Can you work these out from the model? Positions are in its coordinate system, mm. Coordinates: 2 decimals unless noted, no trailing zeros. Order: outer loops, then holes, each group sorted by start corner. A loop starts at its lowest first (then second) coordinate and runs counter-clockwise, first axis right, second up.
```python
from build123d import *

# Parameters (mm, degrees)
SKETCH3_R          = 20.5
SKETCH3_R_2        = 1.5875
EXTRUDE2_DEPTH     = 0.1778
SKETCH5_R          = 1.5
CUT_EXTRUDE1_DEPTH = 29.991923235
CIRPATTERN1_COUNT  = 3


with BuildPart() as part:
    # Sketch3 → Extrude2 (new body)
    with BuildSketch(Plane.XY):
        Circle(SKETCH3_R)
        with Locations((0, 16.5)):
            Circle(SKETCH3_R_2, mode=Mode.SUBTRACT)
        with Locations((14.289419162, -8.25)):
            Circle(SKETCH3_R_2, mode=Mode.SUBTRACT)
        with Locations((-14.289419162, -8.25)):
            Circle(SKETCH3_R_2, mode=Mode.SUBTRACT)
    extrude(amount=EXTRUDE2_DEPTH)

    # Sketch5 → Cut-Extrude1 (cut, through all)
    with BuildSketch(Plane.XY):
        with BuildLine():
            Line((1.5, -20.4450483), (1.5, -16.5))
            ThreePointArc((1.5, -16.5), (0, -18), (-1.5, -16.5))
            Line((-1.5, -16.5), (-1.5, -20.4450483))
            ThreePointArc((-1.5, -20.4450483), (0, -20.5), (1.5, -20.4450483))
        make_face()
        with Locations((0, -16.5)):
            Circle(SKETCH5_R)
    cut_extrude1 = extrude(amount=CUT_EXTRUDE1_DEPTH, mode=Mode.SUBTRACT)

    # CirPattern1: Cut-Extrude1 ×3 about axis, 1 skipped
    cirpattern1_axis = Axis((0, 0, 0.1778), (0, 0, -1))
    add([cut_extrude1.rotate(cirpattern1_axis, i * 360 / CIRPATTERN1_COUNT) for i in range(1, CIRPATTERN1_COUNT) if i not in (1,)], mode=Mode.SUBTRACT)


solid = part.part
```
1. Imagine slicing it at B-B on z = 0.1. Give the number of separate pieces and of enclosed holes in the cut face, then the cut area to 3 significant figures.
Completed:
separate pieces: 1
enclosed holes: 3
area: 1,270 mm2
2. I'm going to push a flat-ended pin straight in: pin 1 (1.9 mm diameter, centred on x = 14.29, y = -8.25, fed in from +Z). Where does the tip first touch, or does it pass through?
Completed:
pin 1: passes through
3. Please list where these lines run through material, in increasing order: probe 1 along Y at (x, z) = (0, 0.1); probe 2 along Y at (x, z) = (13.5, 0.1); probe 3 along X at (y, z) = (-17.5, 0.1).
Completed:
probe 1: y = -15 to 14.91, 18.09 to 20.5
probe 2: y = -15.43 to -9.63, -6.87 to 6.97, 9.53 to 15.43
probe 3: x = -10.68 to -1.5, 1.5 to 10.68
4. Imagine slicing it at A-A on x = 0. Please give me the cut outline in (y, z), then the cut area to 3 significant figures.
Completed:
outline: (-15, 0) - (14.91, 0) - (14.91, 0.18) - (-15, 0.18) - close; (18.09, 0) - (20.5, 0) - (20.5, 0.18) - (18.09, 0.18) - close
area: 5.75 mm2
5. Imagine slicing it at D-D on x = -9. Please give me the cut outline in (y, z), then the cut area to 3 significant figures.
Completed:
outline: (-18.42, 0) - (18.42, 0) - (18.42, 0.18) - (-18.42, 0.18) - close
area: 6.55 mm2
6. Imagine slicing it at C-C on y = 16.5. Please give me the cut outline in (x, z), then the cut area to 3 significant figures.
Completed:
outline: (-12.17, 0) - (-1.59, 0) - (-1.59, 0.18) - (-12.17, 0.18) - close; (1.59, 0) - (12.17, 0) - (12.17, 0.18) - (1.59, 0.18) - close
area: 3.76 mm2
